from build123d import *

# Parameters (mm, degrees)
SKETCH2_W          = 97.871859654
SKETCH2_H          = 113.417127273
CUT_REVOLVE1_ANGLE = 315


with BuildPart() as part:
    # Sketch1 → Revolve2 (revolve)
    with BuildSketch(Plane.XY):
        with BuildLine():
            Line((-69.85, 73.025), (-69.85, 10.954807942))
            Line((-69.85, 10.954807942), (-69.85, 0))
            Line((-69.85, 0), (-67.3735, 0))
            Line((-67.3735, 0), (-65.786, 0))
            Line((-65.786, 0), (-65.786, 9.525))
            Line((-65.786, 9.525), (-63.391760989, 23.103404173))
            ThreePointArc((-63.391760989, 23.103404173), (-60.094186985, 33.816180435), (-51.343091672, 40.820172182))
            ThreePointArc((-51.343091672, 40.820172182), (-27.690740484, 47.825337172), (-3.175, 50.561122579))
            Line((-3.175, 50.561122579), (-3.175, 77.231122579))
            Line((-3.175, 77.231122579), (-5.1435, 77.231122579))
            Line((-5.1435, 77.231122579), (-5.1435, 63.261122579))
            add(Edge.make_bspline(
                [(-5.1435, 63.261122579), (-5.1435, 60.992448788), (-11.791391123, 56.487113553), (-13.98475393, 56.276122579)],
                knots=[0, 0, 0, 0, 1, 1, 1, 1], degree=3))
            ThreePointArc((-13.98475393, 56.276122579), (-32.949086986, 53.181992221), (-51.343091672, 47.625))
            Line((-51.343091672, 47.625), (-66.675, 47.625))
            Line((-66.675, 47.625), (-66.675, 73.025))
            Line((-66.675, 73.025), (-69.85, 73.025))
        make_face()
    revolve(axis=Axis((0, 127.060987048, 0), (0, -1, 0)))

    # Sketch2 → Cut-Revolve1 (revolve, cut)
    with BuildSketch(Plane.XY):
        with Locations((-48.935929827, 30.428788157)):
            Rectangle(SKETCH2_W, SKETCH2_H)
    revolve(axis=Axis((0, 127.060987048, 0), (0, -1, 0)), revolution_arc=CUT_REVOLVE1_ANGLE, mode=Mode.SUBTRACT)


solid = part.part
The listing builds one solid part. Answer for the finished solid, in the listing's coordinates (mm). A direction names the side the tool comes from. Give positions to 0.01 mm unless a question says otherwise; leave off trailing zeros. Write each loop counter-clockwise with the first axis right and the second up, starting at its lowest first coordinate (ties: lowest second). Pieces come first, ordered by that corner, then holes.
Item 1: Section A-A, the plane y = 49 is taken. Write down the section's boundary in (x, z) (3 decimals).
Item 2: Flat-ended cylindrical pins translate along their axes: P1, Ø11.5, axis at x = -62, z = 24.5, coming from the +Y side (3 decimals); P2, Ø2, axis at x = -22.5, z = 11.5, coming from the -Y side; P3, Ø8, axis at y = 60, z = 32, coming from the -X side. Find the tip coordinate at first contact, or state that the pin passes through.
Item 3: Determine the mould class of faces 4 (the flat face through (-63, 73.025, 25)), 5 (the flat face through (-35, 45, 35)), 6 (the cylindrical face through (-61.46, 60.5, 25.85)) for opening direction X: released by +X, released by -X, zero draft, split by the parting line, or undercut.
Item 4: Section B-B, the plane x = -17 is taken. Write down the section's boundary in (y, z), plus the area to 3 significant figures.
Item 5: Find the intervals of material crossed by line 1 along Y through (x, z) = (-60.5, 34) (3 decimals); line 2 along X through (y, z) = (60.5, 2.5); line 3 along X through (y, z) = (31, 41.5), in increasing order.
Item 6: Which of the six approach directions +Z, -Z, +X, -X, +Y, -Y give full straight-line access (tool end or side, diameter ignored) to faces 1 (the cylindrical face through (-4.741, 70.148, 1.994)), 2 (the flat face through (-55, 47.625, 23)), 3 (the cylindrical face through (-60.64, 4.83, 25.51))?
Item 7: Section C-C, the plane y = 5 is taken. Write down the section's boundary in (x, z), plus the area to 3 significant figures.
Completed:
1. outline: (-69.85, 0) - (-66.675, 0) arc R66.675 cw to (-47.146, 47.146) - (-49.391, 49.391) arc R69.85 ccw to start; (-47.521, 0) - (-21.064, 0) arc R21.064 cw to (-14.895, 14.895) - (-33.602, 33.602) arc R47.521 ccw to start
2. P1: stops at y = 73.025
2. P2: stops at y = 48.11
2. P3: stops at x = -63.99
3. face 4: zero draft
3. face 5: released by +X
3. face 6: undercut
4. outline: (48.51, 17) arc R138.66 cw to (49.56, 0) - (55.95, 0) arc R145.06 ccw to (54.95, 17) - close
4. area: 109 mm2
5. line 1: y = 0 to 73.025
5. line 2: x = -69.81 to -66.63, -6.47 to -2.5
5. line 3: x = -56.19 to -45.63
6. face 1: +Z, +Y
6. face 2: +Y
6. face 3: -Z, +X, -Y
7. outline: (-69.85, 0) - (-65.79, 0) arc R65.79 cw to (-46.52, 46.52) - (-49.39, 49.39) arc R69.85 ccw to start
7. area: 216 mm2
